```python
from build123d import *

# Parameters (mm, degrees)
F0_W     = 50
F0_H     = 80
F1_DEPTH = 25
F2_T     = -2.5
F3_W     = 2.5
F3_H     = 17.840053
F3_H_2   = 18.443981
F4_DEPTH = 60
F6_D     = 10


with BuildPart() as f1:
    # F0 (on Top) → F1 (new body)
    with BuildSketch(Plane.XY):
        Rectangle(F0_W, F0_H)
    extrude(amount=F1_DEPTH)

    # F2
    f2_openings = [f1.faces().sort_by_distance(p)[0] for p in [
        (0, 0, 25),
    ]]
    offset(amount=F2_T, openings=f2_openings)

    # F3 (on face) → F4 (join)
    with BuildSketch(Plane.XY.offset(25)):
        with Locations((-23.75, -0.518573)):
            Rectangle(F3_W, F3_H)
        with Locations((23.75, -0.216609)):
            Rectangle(F3_W, F3_H_2)
    extrude(amount=F4_DEPTH)

    # F6 (through all)
    with Locations(Plane.YZ.offset(25)):
        with Locations((0, 77.299073)):
            Hole(F6_D / 2)


solid = f1.part
```
The listing builds one solid part. Answer for the finished solid, in the listing's coordinates (mm). A direction names the side the tool comes from. Round coordinates to 2 decimals unless told otherwise and drop trailing zeros. Loops run counter-clockwise (first coordinate to the right, second up) from the corner with the lowest first, then second, coordinate; pieces in that order, holes last.
Q1. Section A-A, the plane y = 0 is taken. Determine the outline of the cut face in (x, z).
Q2. Given pin 1 Ø2 at (x, z) = (24, 41.5) entering from -Y; pin 2 Ø22.5 at (x, y) = (10, 11.5) entering from +Z; pin 3 Ø2 at (x, z) = (-24, 69) entering from +Y, each flat-ended and moving along its own axis, determine where each tip first touches the part or whether it passes through.
Q3. For a pull along Y with two mould halves and no side action, classify faces 5 (the face through (-24, 0, 85)), 6 (the face through (22.5, -1, 34)), 7 (the face through (-24, 8.401, 55)) as released by +Y, released by -Y, zero draft, split by the parting line, or undercut.
Q4. Section C-C, the plane x = -20 is taken. Determine the outline of the cut face in (y, z).
Q5. Section B-B, the plane z = 46 is taken. Determine the outline of the cut face in (x, y), then the cut area to 3 significant figures.
Q6. Which of the six approach directions +Z, -Z, +X, -X, +Y, -Y give full straight-line access (tool end or side, diameter ignored) to faces 1 (the face through (24, 9.005, 55)), 2 (the face through (0, 37.5, 14)), 3 (the face through (25, -1, 23)), 4 (the face through (24, -9.439, 55))?
Q7. Find the intervals of material crossed by line 1 (X direction, y = 6, z = 50); line 2 (Z direction, x = 23, y = 0); line 3 (Y direction, x = 19, z = 17.5), in increasing order.
Q8. Section D-D, the plane z = 15 is taken. Determine the outline of the cut face in (x, y).
Completed:
1. outline: (-25, 0) - (25, 0) - (25, 72.3) - (22.5, 72.3) - (22.5, 2.5) - (-22.5, 2.5) - (-22.5, 72.3) - (-25, 72.3) - close; (-25, 82.3) - (-22.5, 82.3) - (-22.5, 85) - (-25, 85) - close; (22.5, 82.3) - (25, 82.3) - (25, 85) - (22.5, 85) - close
2. pin 1: stops at y = -9.44
2. pin 2: stops at z = 2.5
2. pin 3: stops at y = 8.4
3. face 5: zero draft
3. face 6: undercut
3. face 7: released by +Y
4. outline: (-40, 0) - (40, 0) - (40, 25) - (37.5, 25) - (37.5, 2.5) - (-37.5, 2.5) - (-37.5, 25) - (-40, 25) - close
5. outline: (-25, -9.44) - (-22.5, -9.44) - (-22.5, 8.4) - (-25, 8.4) - close; (22.5, -9.44) - (25, -9.44) - (25, 9.01) - (22.5, 9.01) - close
5. area: 90.7 mm2
6. face 1: +Z, +X, -X, +Y
6. face 2: +Z
6. face 3: +Z, -Z, +X, +Y, -Y
6. face 4: +Z, +X, -X, -Y
7. line 1: x = -25 to -22.5, 22.5 to 25
7. line 2: z = 0 to 72.3, 82.3 to 85
7. line 3: y = -40 to -37.5, 37.5 to 40
8. outline: (-25, -40) - (25, -40) - (25, 40) - (-25, 40) - close; hole (-22.5, -37.5) - (22.5, -37.5) - (22.5, 37.5) - (-22.5, 37.5) - close
